Build history of the part. All positions in model axes, mm. Face numbers are marked on the shaded views. A direction names the side the tool comes from. Round coordinates to 2 decimals unless told otherwise and drop trailing zeros. Order: outer loops, then holes, each group sorted by start corner. A loop starts at its lowest first (then second) coordinate and runs counter-clockwise, first axis right, second up. Notation, with made-up numbers: (1, 71) -> (15, 71) arc R9 cw to (15, 86) -> close; hole circle Ø9 at (-9, 3). An arc over 180 degrees is marked (long way). Use a Markdown table: item, result. Add a question column.
Item 1: Two-plate mould, pull along Y, no slides. Class the marked faces 4, 5 and 6: released by +Y, released by -Y, zero draft, split by the parting line, or undercut.
Item 2: Slice it at A-A, the plane z = 56. Give the cut face in (x, y), plus the area to 3 significant figures.
Item 3: Pin check, flat tips, straight feed: pin 1 (8 mm diameter, centred on y = 27, z = 202.5, fed in from -X); pin 2 (1 mm diameter, centred on x = 22, z = 274, fed in from -Y); pin 3 (6 mm diameter, centred on x = -16, y = 10, fed in from +Z). Stop position of each tip, or through.
Item 4: 3-axis set-ups, long thin cutter, end or side, ignore diameter. For the marked faces 1, 2 and 3: which of +Z, -Z, +X, -X, +Y, -Y reach the whole face in a straight line?
Item 5: Slice it at B-B, the plane z = 208. Give the cut face in (x, y), plus the area to 3 significant figures.
Item 6: Probe L1, parallel to Y at x = 0, z = 114; L2, parallel to Y at x = 0, z = 213.5; L3, parallel to Z at x = 43, y = -28.5. List the from-to ranges inside material, lowest first.
from build123d import *

# Parameters (mm, degrees)
F0_R     = 38.1
F1_DEPTH = 114.3
F2_R     = 30.48
F3_DEPTH = 215.9
F5_D     = 48.514
F5_DEPTH = 304.8
F5_TIP   = 14.5750760358
F6_W     = 114.3
F6_H     = 76.2
F7_DEPTH = 6.35


with BuildPart() as f1:
    # F0 (on Top) → F1 (new body)
    with BuildSketch(Plane.XY):
        Circle(F0_R)
    extrude(amount=F1_DEPTH)

    # F2 (on face) → F3 (join)
    with BuildSketch(Plane.XY.offset(114.3)):
        Circle(F2_R)
    extrude(amount=F3_DEPTH)

    # F5
    with Locations(Plane.XY.offset(330.2)):
        with Locations((0, 0)):
            Hole(F5_D / 2, depth=F5_DEPTH)
            with Locations((0, 0, -(F5_DEPTH + F5_TIP / 2))):  # 118° drill point
                Cone(0, F5_D / 2, F5_TIP, mode=Mode.SUBTRACT)

    # F6 (on Top) → F7 (join)
    with BuildSketch(Plane.XY):
        Rectangle(F6_W, F6_H)
    extrude(amount=-F7_DEPTH)


solid = f1.part
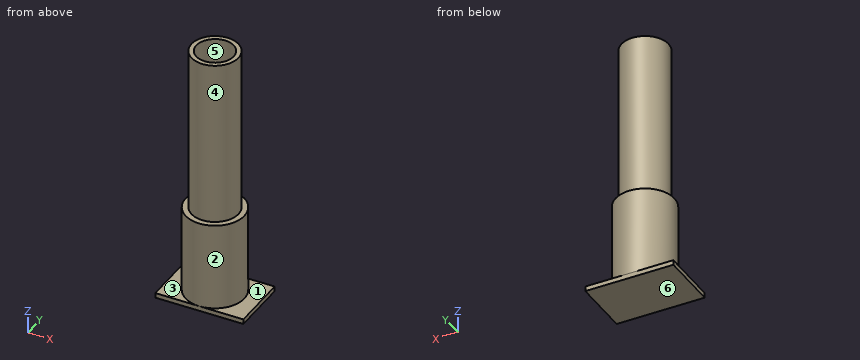
Check sheet entries:
| question | item | result |
|---|---|---|
| 1 | face 4 | split by the parting line |
| 1 | face 5 | undercut |
| 1 | face 6 | zero draft |
| 2 | outline | circle Ø76.2 at (0, 0); hole circle Ø48.51 at (0, 0) |
| 2 | area | 2,710 mm2 |
| 3 | pin 1 | x = -20 |
| 3 | pin 2 | y = -21.61 |
| 3 | pin 3 | z = 23.96 |
| 4 | face 1 | +Z, +X |
| 4 | face 2 | +Z |
| 4 | face 3 | +Z, -X |
| 5 | outline | circle Ø60.96 at (0, 0); hole circle Ø48.51 at (0, 0) |
| 5 | area | 1,070 mm2 |
| 6 | L1 | -38.1 to -24.26, 24.26 to 38.1 |
| 6 | L2 | -30.48 to -24.26, 24.26 to 30.48 |
| 6 | L3 | -6.35 to 0 |
